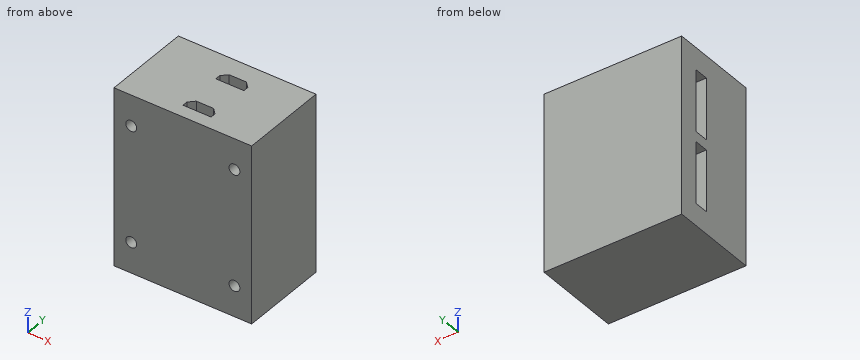
Autodesk Inventor part; units mm, degrees
ref_plane "YZ Plane" through (0, 0, 0) normal (1, 0, 0) x (0, 1, 0)
ref_plane "XZ Plane" through (0, 0, 0) normal (0, 1, 0) x (-1, 0, 0)
ref_plane "XY Plane" through (0, 0, 0) normal (0, 0, 1) x (1, 0, 0)
sketch "Sketch1" plane through (0, 0, 0) normal (0, 1, 0) x (-1, 0, 0)
  line L0 (0, 0) -> (38, 0)
  line L1 (38, 0) -> (38, -49)
  line L2 (38, -49) -> (0, -49)
  line L3 (0, -49) -> (0, 0)
  dimension "d0" = 38
  dimension "d1" = 49
extrude "Extrusion1" add sketch "Sketch1" along normal blind 24.5
sketch "Sketch3" plane through (-38, 0, -49) normal (-1, 0, 0) x (0, 0, 1)
  line L0 (0, 0) -> (0, 24.5)
  line L1 (0, 0) -> (0, 15.1)
  line L2 (0, 15.1) -> (6.1, 15.1)
  line L3 (6.1, 15.1) -> (23.1, 15.1)
  line L4 (23.1, 15.1) -> (23.1, 19)
  line L5 (23.1, 19) -> (6.1, 19)
  line L6 (6.1, 19) -> (6.1, 15.1)
  line L7 (0, 0) -> (49, 0)
  line L8 (0, 0) -> (49, 0)
  line L9 (24.5, 0) -> (24.5, -2.7502)
  line L10 (49, 15.1) -> (42.9, 15.1)
  line L11 (42.9, 15.1) -> (25.9, 15.1)
  line L12 (25.9, 15.1) -> (25.9, 19)
  line L13 (25.9, 19) -> (42.9, 19)
  line L14 (42.9, 19) -> (42.9, 15.1)
  dimension "d8" = 15.1
  dimension "d9" = 6.1
  dimension "d10" = 17
  dimension "d11" = 3.9
extrude "Extrusion2" cut sketch "Sketch3" against normal blind 15
sketch "Sketch4" plane through (-38, 0, 0) normal (0, 0, 1) x (1, 0, 0)
  line L0 (0, 0) -> (0, 24.5)
  line L1 (0, 24.5) -> (16.4, 24.5)
  line L2 (0, 24.5) -> (38, 24.5)
  line L3 (16.4, 24.5) -> (16.4, 16.15)
  line L4 (16.4, 16.15) -> (24.15, 16.15)
  line L5 (24.15, 16.15) -> (24.15, 19.15)
  line L6 (24.15, 19.15) -> (16.4, 19.15)
  line L7 (16.4, 19.15) -> (16.4, 16.15)
  line L8 (16.4, 16.15) -> (16.4, 3.65)
  line L9 (16.4, 3.65) -> (24.15, 3.65)
  line L10 (24.15, 3.65) -> (24.15, 6.65)
  line L11 (24.15, 6.65) -> (16.4, 6.65)
  line L12 (16.4, 6.65) -> (16.4, 3.65)
  point P0 (38, 0)
  point P1 (16.4, 6.65)
  point P2 (16.4, 19.15)
  dimension "d14" = 16.4
  dimension "d15" = 8.35
  dimension "d16" = 7.75
  dimension "d17" = 3
  dimension "d18" = 12.5
  dimension "d19" = 7.75
  dimension "d20" = 3
extrude "Extrusion3" cut sketch "Sketch4" against normal blind 15
chamfer "Chamfer1" distance 1.5 angle 45 4 edges at (-13.85, 19.15, -7.5) (-13.85, 6.65, -7.5) (-21.6, 19.15, -7.5) (-21.6, 6.65, -7.5)
sketch "Sketch5" plane through (0, 0, 0) normal (0, -1, 0) x (1, 0, 0)
  line L0 (-38, 0) -> (0, 0)
  line L1 (0, 0) -> (-4.75, 0)
  line L2 (-4.75, 0) -> (-4.75, -8.5)
  line L3 (-4.75, -8.5) -> (-4.75, -40.5)
  line L4 (-4.75, -40.5) -> (-33.25, -40.5)
  line L5 (-33.25, -40.5) -> (-33.25, -8.5)
  line L6 (-38, -6.1) -> (-23, -6.1)
  circle A0 centre (-33.25, -40.5) radius 1.5
  circle A1 centre (-4.75, -40.5) radius 1.5
  circle A2 centre (-4.75, -8.5) radius 1.5
  circle A3 centre (-33.25, -8.5) radius 1.5
  dimension "d26" = 4.75
  dimension "d27" = 8.5
  dimension "d28" = 32
  dimension "d29" = 28.5
  dimension "d30" = 3
  dimension "d31" = 3
  dimension "d32" = 3
  dimension "d33" = 3
extrude "Extrusion4" cut sketch "Sketch5" against normal blind 10
properties part number "Contactile Communication Hub"
CAD build for the part. Positions are in the model's coordinates, mm. Round coordinates to 2 decimals unless told otherwise and drop trailing zeros. Order: outer loops, then holes, each group sorted by start corner. A loop starts at its lowest first (then second) coordinate and runs counter-clockwise, first axis right, second up. Notation, with made-up numbers: (39, 71) -> (72, 71) arc R22 cw to (72, 90) -> close; hole circle Ø9 at (71, 77.25). An arc over 180 degrees is marked (long way). Write item = value, one per line.
(1) Cut at C-C (y = 2.25). Write the cut outline in (x, z).
Answers follow:
outline = (-38, -49) -> (0, -49) -> (0, 0) -> (-38, 0) -> close; hole circle Ø3 at (-33.25, -40.5); hole circle Ø3 at (-33.25, -8.5); hole circle Ø3 at (-4.75, -40.5); hole circle Ø3 at (-4.75, -8.5)
(2) Cut at B-B (x = -27). Write the cut outline in (y, z), plus the area to 3 significant figures.
Answers follow:
outline = (0, -49) -> (24.5, -49) -> (24.5, 0) -> (0, 0) -> close; hole (15.1, -42.9) -> (19, -42.9) -> (19, -25.9) -> (15.1, -25.9) -> close; hole (15.1, -23.1) -> (19, -23.1) -> (19, -6.1) -> (15.1, -6.1) -> close
area = 1,070 mm²
(3) Flat gauge pins, fed straight in: P1, Ø0.9, axis at x = -19, y = 5.5, coming from the +Z side; P2, Ø1.5, axis at x = -5, z = -9, coming from the -Y side. Where does each tip first touch, or does it go through?
Answers follow:
P1 = -15
P2 = 10
(4) Drill centre lines: L1, parallel to Y at x = -17, z = -4.5; L2, parallel to X at y = 5.25, z = -40.5; L3, parallel to Z at x = -33.25, y = 4. Where is each one in solid material? Low to high.
Answers follow:
L1 = 0 to 3.65, 6.65 to 16.15, 19.15 to 24.5
L2 = -38 to -34.75, -31.75 to -6.25, -3.25 to 0
L3 = -49 to -42, -39 to -10, -7 to 0
(5) Cut at D-D (x = -4.75). Write the cut outline in (y, z), plus the area to 3 significant figures.
Answers follow:
outline = (0, -49) -> (24.5, -49) -> (24.5, 0) -> (0, 0) -> (0, -7) -> (10, -7) -> (10, -10) -> (0, -10) -> (0, -39) -> (10, -39) -> (10, -42) -> (0, -42) -> close
area = 1,140 mm²
(6) Cut at A-A (z = -4). Write the cut outline in (x, y).
Answers follow:
outline = (-38, 0) -> (0, 0) -> (0, 24.5) -> (-38, 24.5) -> close; hole (-21.6, 3.65) -> (-13.85, 3.65) -> (-13.85, 5.15) -> (-15.35, 6.65) -> (-20.1, 6.65) -> (-21.6, 5.15) -> close; hole (-21.6, 16.15) -> (-13.85, 16.15) -> (-13.85, 17.65) -> (-15.35, 19.15) -> (-20.1, 19.15) -> (-21.6, 17.65) -> close
